Verification items for the finished model (mm, model axes). Face numbers are marked on the shaded views. A direction names the side the tool comes from. Give positions to 0.01 mm unless a question says otherwise; leave off trailing zeros. Loops run counter-clockwise (first coordinate to the right, second up) from the corner with the lowest first, then second, coordinate; pieces in that order, holes last. Notation, with made-up numbers: (-28.75, -24.75) - (-21.75, -24.75) arc R18 cw to (-21.75, -0.75) - close; hole circle Ø2 at (-16, 68). An arc over 180 degrees is marked (long way). Put each result on its own line as item: value. Start each with the question number.
```python
from build123d import *

# Parameters (mm, degrees)
SKETCH_1_W          = 120
SKETCH_1_H          = 80
EXTRUDE_1_DEPTH     = 150
SHELL_1_T           = -5
EXTRUDE_2_DEPTH     = 5
SKETCH_3_R          = 15
CUT_EXTRUDE_1_DEPTH = 10000


with BuildPart() as part:
    # 草图1 → 凸台-拉伸1 (new body)
    with BuildSketch(Plane.XY):
        Rectangle(SKETCH_1_W, SKETCH_1_H)
    extrude(amount=EXTRUDE_1_DEPTH)

    # 抽壳1
    shell_1_openings = [part.faces().sort_by_distance(p)[0] for p in [
        (0, -40, 75),
    ]]
    offset(amount=SHELL_1_T, openings=shell_1_openings, kind=Kind.INTERSECTION)

    # 草图2 → 凸台-拉伸2 (add)
    with BuildSketch(Plane.XZ.offset(40)):
        Polygon((-60, 150), (-70, 150), (-70, -10), (70, -10), (70, 150), (60, 150), (60, 0), (-60, 0), align=None)
    extrude(amount=-EXTRUDE_2_DEPTH)

    # 草图3 → 切除-拉伸1 (cut)
    with BuildSketch(Plane(origin=(0, 0, 0), x_dir=(-1, 0, 0), z_dir=(0, 0, -1))):
        with Locations((0, -5)):
            Circle(SKETCH_3_R)
    extrude(amount=-CUT_EXTRUDE_1_DEPTH, mode=Mode.SUBTRACT)


solid = part.part
```
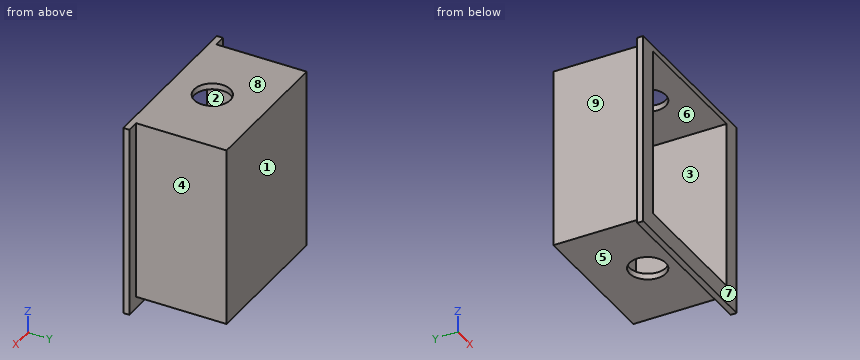
1) Section check C-C, the plane y = -23. Enter the section's corners in (x, z), plus the area to 3 significant figures.
2) Set-up check for the marked faces 5, 6, 7, 8 and 9: record each of +Z, -Z, +X, -X, +Y, -Y from which the full face is reachable in a straight line by a thin tool's end or side.
3) Depth check by flat-ended pin: P1, Ø12, axis at y = -6, z = 125, coming from the -X side; P2, Ø6, axis at x = 13, y = -21, coming from the -Z side; P3, Ø3, axis at x = -45.5, z = 33, coming from the -Y side; P4, Ø18, axis at x = 0, y = -5, coming from the -Z side. Enter the tip coordinate at first touch or a pass-through.
4) Section check D-D, the plane x = 35.5. Enter the section's corners in (y, z), plus the area to 3 significant figures.
5) Scan lines: line 1 along Z through (x, y) = (37, -12.5); line 2 along Y through (x, z) = (0, 1.6); line 3 along X through (y, z) = (-33, 110). Record each from-to range of solid material in increasing order. Write a range as from..to.
6) Draft check along X on the marked faces 1, 2, 3 and 4. Enter one of: pulls with the +X half, pulls with the -X half, needs draft (parallel to the pull), parting line crosses it, or undercut.
7) Section check B-B, the plane x = 0. Enter the section's corners in (y, z).
8) Section check A-A, the plane y = -5. Enter the section's corners in (x, z), plus the area to 3 significant figures.
Results are:
1. outline: (-60, 0) - (60, 0) - (60, 150) - (-60, 150) - close; hole (-55, 5) - (55, 5) - (55, 145) - (-55, 145) - close
1. area: 2,600 mm2
2. face 5: -Z, +X, -X, +Y
2. face 6: -Y
2. face 7: +Z, -Z, +X, -X, -Y
2. face 8: +Z, +X, -X, +Y, -Y
2. face 9: +Z, -Z, -X, +Y
3. P1: stops at x = -60
3. P2: stops at z = 0
3. P3: stops at y = 35
3. P4: passes through
4. outline: (-40, -10) - (-35, -10) - (-35, 0) - (40, 0) - (40, 150) - (-40, 150) - (-40, 145) - (35, 145) - (35, 5) - (-40, 5) - close
4. area: 1,550 mm2
5. line 1: z = 0..5, 145..150
5. line 2: y = -40..-20, 10..40
5. line 3: x = -60..-55, 55..60
6. face 1: needs draft
6. face 2: undercut
6. face 3: undercut
6. face 4: pulls with the +X half
7. outline: (-40, -10) - (-35, -10) - (-35, 0) - (-20, 0) - (-20, 5) - (-40, 5) - close; (-40, 145) - (-20, 145) - (-20, 150) - (-40, 150) - close; (10, 0) - (40, 0) - (40, 150) - (10, 150) - (10, 145) - (35, 145) - (35, 5) - (10, 5) - close
8. outline: (-60, 0) - (-15, 0) - (-15, 5) - (-55, 5) - (-55, 145) - (-15, 145) - (-15, 150) - (-60, 150) - close; (15, 0) - (60, 0) - (60, 150) - (15, 150) - (15, 145) - (55, 145) - (55, 5) - (15, 5) - close
8. area: 2,300 mm2
